The model under review builds one solid part; all positions refer to its coordinate system, in mm. A direction names the side the tool comes from. Round coordinates to 2 decimals unless told otherwise and drop trailing zeros. Loops run counter-clockwise (first coordinate to the right, second up) from the corner with the lowest first, then second, coordinate; pieces in that order, holes last. Notation, with made-up numbers: M 82,75.25 L 93,75.25 A11 ccw 93,89.25 Z; hole C -19.75,-15 d4. An arc over 180 degrees is marked long. Return JSON: item names as keys, results as strings. Group by question number.
Q1. Consider section B-B (y = 2.75). State the section outline as (x, z) points, and give its area (3 significant figures).
Q2. Consider section A-A (z = 3.7). State the section outline as (x, y) points, and give its area (3 significant figures).
Q3. For faces 5 (the face through (3.63, 0.64, 2.99)), 6 (the face through (2.5, 5.5, 3)), 7 (the face through (2.5, 6.5, 3)), 8 (the face through (-4, 5, 3)), 9 (the face through (4.141, 3, 3)), list the 3-axis set-ups (+Z, -Z, +X, -X, +Y, -Y) from which the entire face can be reached by the end or side of a thin tool; tool diameter is ignored.
Q4. Consider section D-D (y = -1.5). State the section outline as (x, z) points, and give its area (3 significant figures).
Q5. Clearance check with flat-ended pins moving along their axes: pin 1 Ø2 at (y, z) = (2, 2.5) entering from -X; pin 2 Ø2 at (y, z) = (3, 3.5) entering from +X; pin 3 Ø1 at (y, z) = (-3.5, 3.5) entering from -X; pin 4 Ø3 at (x, y) = (0.5, -0.5) entering from +Z. State where each tip first meets the part, or that it passes through.
Q6. To check wall thickness, follow line 1 along X through (y, z) = (4.5, 3.8); line 2 along Z through (x, y) = (-0.25, -3); line 3 along X through (y, z) = (-2.75, 3.6). State the ranges of each line that lie inside material, in increasing order.
Q7. Consider section C-C (x = -1.5). State the section outline as (y, z) points.
Q8. Draft analysis for pull direction Y (two halves, no side actions). For faces 1 (the face through (2.63, 0.6, 2.99)), 2 (the face through (4, 5, 3)), 3 (the face through (3, 3, 4)), 4 (the face through (2.65, -0.58, 2.99)), state which applies: pulls with the +Y half, pulls with the -Y half, needs draft (parallel to the pull), parting line crosses it, or undercut.
from build123d import *

# Parameters (mm, degrees)
F0_W     = 10
F0_H     = 16
F1_DEPTH = 2
F3_DEPTH = 2


with BuildPart() as f1:
    # F0 (on Top) → F1 (new body)
    with BuildSketch(Plane.XY):
        Rectangle(F0_W, F0_H)
    extrude(amount=F1_DEPTH)

    # F2 (on face) → F3 (join)
    with BuildSketch(Plane.XY.offset(2)):
        Polygon((0, 7), (-2, 7), (-3, 6), (-2, 5), (0, 5), (2, 5), (3, 6), (2, 7), align=None)
        Polygon((-2.141421, 4.858579), (-3.141421, 5.858579), (-4.141421, 4.858579), (-4.141421, 1.150722), (-3.137452, 0.145399), (-2.141421, 1.03352), align=None)
        Polygon((4.141421, 4.858579), (3.141421, 5.858579), (2.141421, 4.858579), (2.141421, 1.03352), (3.137452, 0.145399), (4.141421, 1.150722), align=None)
        Polygon((3.137452, -0.145399), (2.141421, -1.03352), (2.141421, -4.858579), (3.141421, -5.858579), (4.141421, -4.858579), (4.141421, -1.150722), align=None)
    extrude(amount=F3_DEPTH)


solid = f1.part
Values:
{
 "1": {"outline": "M -5,0 L 5,0 L 5,2 L 4.14,2 L 4.14,4 L 2.14,4 L 2.14,2 L -2.14,2 L -2.14,4 L -4.14,4 L -4.14,2 L -5,2 Z", "area": "28.0 mm2"},
 "2": {"outline": "M -4.14,1.15 L -3.14,0.15 L -2.14,1.03 L -2.14,4.86 L -3.14,5.86 L -4.14,4.86 Z; M -3,6 L -2,5 L 2,5 L 3,6 L 2,7 L -2,7 Z; M 2.14,-4.86 L 3.14,-5.86 L 4.14,-4.86 L 4.14,-1.15 L 3.14,-0.15 L 2.14,-1.03 Z; M 2.14,1.03 L 3.14,0.15 L 4.14,1.15 L 4.14,4.86 L 3.14,5.86 L 2.14,4.86 Z", "area": "38.4 mm2"},
 "3": {"face 5": "+Z, +X", "face 6": "+Z", "face 7": "+Z, +X, +Y", "face 8": "+Z, -X, +Y", "face 9": "+Z, +X, +Y, -Y"},
 "4": {"outline": "M -5,0 L 5,0 L 5,2 L 4.14,2 L 4.14,4 L 2.14,4 L 2.14,2 L -5,2 Z", "area": "24.0 mm2"},
 "5": {"pin 1": "stops at x = -5", "pin 2": "stops at x = 4.14", "pin 3": "stops at x = 2.14", "pin 4": "stops at z = 2"},
 "6": {"line 1": "x = -4.14 to -2.14, 2.14 to 4.14", "line 2": "z = 0 to 2", "line 3": "x = 2.14 to 4.14"},
 "7": {"outline": "M -8,0 L 8,0 L 8,2 L 7,2 L 7,4 L 5,4 L 5,2 L -8,2 Z"},
 "8": {"face 1": "undercut", "face 2": "pulls with the +Y half", "face 3": "needs draft", "face 4": "undercut"}
}
